Source: CAD feature listing. Evaluate the final solid. Frame: model axes, mm. Face numbers are marked on the shaded views. Give positions to 0.01 mm unless a question says otherwise; leave off trailing zeros. Order: outer loops, then holes, each group sorted by start corner. A loop starts at its lowest first (then second) coordinate and runs counter-clockwise, first axis right, second up. Notation, with made-up numbers: M -31.5,13.25 L -9.5,13.25 A18 ccw -9.5,47.25 Z; hole C 31,86.25 d1. An arc over 180 degrees is marked long. Use CSV: the item, a comma, the result in double quotes. Start each with the question number.
Item 1: Section query D-D on x = 22. Return loops of the section in (y, z), and give its area (3 significant figures).
Item 2: First-contact query: pin 1 (1.8 mm diameter, centred on x = -52, y = 6.5, fed in from +Z); pin 2 (4 mm diameter, centred on y = 14, z = 1.5, fed in from -X); pin 3 (5.5 mm diameter, centred on x = -49.5, y = 6, fed in from -Z); pin 4 (1.8 mm diameter, centred on y = 3.5, z = 7, fed in from -X). Flat tips, straight axial feed; report the tip coordinate or a pass-through.
Item 3: Section query A-A on x = -36. Return loops of the section in (y, z).
Item 4: Section query C-C on y = 4. Return loops of the section in (x, z).
Item 5: Section query B-B on z = 7.5. Return loops of the section in (x, y).
Item 6: Ray query, probe 1 along X at (y, z) = (6.5, 2); probe 2 along Y at (x, z) = (-21, 5.6); probe 3 along Y at (x, z) = (-43.5, 9.5). Return the intervals inside material, ascending. Write a range as from..to.
Item 7: Pull-direction query (X, two-part tool) for the marked faces 1, 2 and 3; classes: +X half, -X half, draft (parallel to the pull), parting line (faces both ways), or undercut.
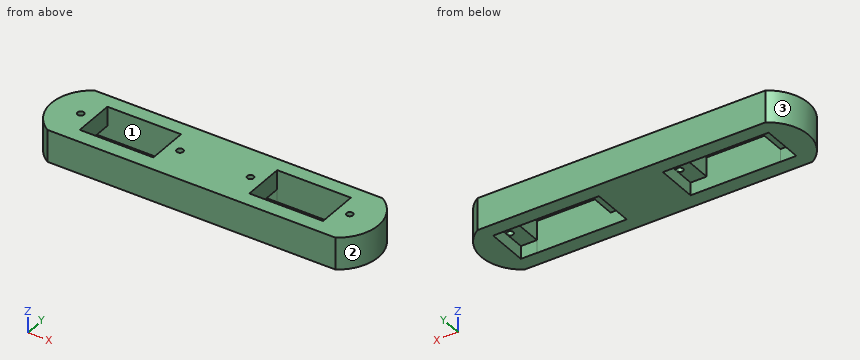
from build123d import *

# Parameters (mm, degrees)
EXTRUDE_2_DEPTH     = 10
SKETCH_2_W          = 5
SKETCH_2_H          = 12.958862493
CUT_EXTRUDE_2_DEPTH = 4
SKETCH_3_W          = 23
SKETCH_3_H          = 13
SKETCH_3_H_2        = 12.917724986
CUT_EXTRUDE_4_DEPTH = 11
SKETCH_4_R          = 1
CUT_EXTRUDE_5_DEPTH = 11


with BuildPart() as part:
    # 草图1 → 凸台-拉伸2 (new body)
    with BuildSketch(Plane.XY):
        with BuildLine():
            Line((-55, 17.378078065), (35, 17.378078065))
            ThreePointArc((35, 17.378078065), (41.07179677, 6.378078065), (35, -4.621921935))
            Line((35, -4.621921935), (-55, -4.621921935))
            ThreePointArc((-55, -4.621921935), (-61.07179677, 6.378078065), (-55, 17.378078065))
        make_face()
    extrude(amount=EXTRUDE_2_DEPTH)

    # 草图2 → 切除-拉伸2 (cut)
    with BuildSketch(Plane(origin=(0, 0, 0), x_dir=(-1, 0, 0), z_dir=(0, 0, -1))):
        with Locations((-30.5, 6.520568754)):
            Rectangle(SKETCH_2_W, SKETCH_2_H)
        with Locations((-2.5, 6.479431247)):
            Rectangle(SKETCH_2_W, SKETCH_2_H)
        with Locations((22.5, 6.520568754)):
            Rectangle(SKETCH_2_W, SKETCH_2_H)
        with Locations((50.5, 6.479431247)):
            Rectangle(SKETCH_2_W, SKETCH_2_H)
    extrude(amount=-CUT_EXTRUDE_2_DEPTH, mode=Mode.SUBTRACT)

    # 草图3 → 切除-拉伸4 (cut, through all)
    with BuildSketch(Plane(origin=(0, 0, 0), x_dir=(-1, 0, 0), z_dir=(0, 0, -1))):
        with Locations((-16.5, 6.5)):
            Rectangle(SKETCH_3_W, SKETCH_3_H)
        with Locations((36.5, 6.5)):
            Rectangle(SKETCH_3_W, SKETCH_3_H_2)
    extrude(amount=-CUT_EXTRUDE_4_DEPTH, mode=Mode.SUBTRACT)

    # 草图4 → 切除-拉伸5 (cut, through all)
    with BuildSketch(Plane(origin=(0, 0, 0), x_dir=(-1, 0, 0), z_dir=(0, 0, -1))):
        with Locations((-32, 6.5)):
            Circle(SKETCH_4_R)
        with Locations((-1, 6.5)):
            Circle(SKETCH_4_R)
        with Locations((21, 6.5)):
            Circle(SKETCH_4_R)
        with Locations((52, 6.5)):
            Circle(SKETCH_4_R)
    extrude(amount=-CUT_EXTRUDE_5_DEPTH, mode=Mode.SUBTRACT)


solid = part.part
Verdict:
1,outline,"M -4.62,0 L 0,0 L 0,10 L -4.62,10 Z; M 13,0 L 17.38,0 L 17.38,10 L 13,10 Z"
1,area,"90.0 mm2"
2,pin 1,"through"
2,pin 2,"x = -59.79"
2,pin 3,"z = 4"
2,pin 4,"x = -60.92"
3,outline,"M -4.62,0 L 0.04,0 L 0.04,10 L -4.62,10 Z; M 12.96,0 L 17.38,0 L 17.38,10 L 12.96,10 Z"
4,outline,"M -60.85,0 L -53,0 L -53,4 L -48,4 L -48,10 L -60.85,10 Z; M -25,4 L -20,4 L -20,0 L 0,0 L 0,4 L 5,4 L 5,10 L -25,10 Z; M 28,4 L 33,4 L 33,0 L 40.85,0 L 40.85,10 L 28,10 Z"
5,outline,"M -55,-4.62 L 35,-4.62 A13 ccw 35,17.38 L -55,17.38 A13 ccw Z; hole C -52,6.5 d2; hole M -48,0.04 L -25,0.04 L -25,12.96 L -48,12.96 Z; hole C -21,6.5 d2; hole C 1,6.5 d2; hole M 5,0 L 28,0 L 28,13 L 5,13 Z; hole C 32,6.5 d2"
6,probe 1,"-61.07..-53, -20..0, 33..41.07"
6,probe 2,"-4.62..5.5, 7.5..17.38"
6,probe 3,"-4.62..0.04, 12.96..17.38"
7,face 1,"undercut"
7,face 2,"+X half"
7,face 3,"-X half"
